from build123d import *

# Parameters (mm, degrees)
F1_DEPTH = 3
F2_W     = 261
F2_H     = 166
F2_R     = 3
F3_DEPTH = 3
F4_R     = 4.99999


# Not quite as in the source:
# - a fillet or chamfer is up to 0.001 mm smaller than in the source, because OpenCascade refuses the exact size


with BuildPart() as f1:
    # F0 (on Front) → F1 (new body)
    with BuildSketch(Plane.XZ):
        Polygon((170, -120), (170, 120), (-170, 120), (-170, -120), (-165, -120), (-165, -110), (-159.5, -110), (-159.5, -120), (159.5, -120), (159.5, -110), (165, -110), (165, -120), align=None)
    extrude(amount=F1_DEPTH)

    # F2 (on face) → F3 (cut, through all)
    with BuildSketch(Plane.XZ.offset(3)):
        Rectangle(F2_W, F2_H)
        with Locations((0, -112)):
            Circle(F2_R)
    extrude(amount=-F3_DEPTH, mode=Mode.SUBTRACT)

    # F4 (radius 5 in the source; OpenCascade refuses exactly that, so slightly less here)
    f4_edges = [f1.edges().sort_by_distance(p)[0] for p in [
        (-170, -1.5, 120),
        (170, -1.5, 120),
        (170, -1.5, -120),
        (-170, -1.5, -120),
    ]]
    fillet(f4_edges, radius=F4_R)


solid = f1.part
For this review, take the finished solid that the model builds, in its own axes (mm). Round coordinates to 2 decimals unless told otherwise and drop trailing zeros. Write each loop counter-clockwise with the first axis right and the second up, starting at its lowest first coordinate (ties: lowest second). Pieces come first, ordered by that corner, then holes. Notation, with made-up numbers: M 71,73 L 91,73 A19 cw 91,103 Z; hole C 80.25,10.5 d8. An arc over 180 degrees is marked long. Write item = value, one per line. Start each with the question number.
(1) We need section B-B (z = -57). Give the boundary of the cut face in (x, y).
(2) We need section C-C (y = -0.6). Give the number of separate pieces and of enclosed holes in the cut face, then the cut area to 3 significant figures.
(3) Clearance check with flat-ended pins moving along their axes: pin 1 Ø1.5 at (x, y) = (161.5, -1) entering from -Z; pin 2 Ø0.9 at (y, z) = (-1.5, -117) entering from +X; pin 3 Ø5 at (x, z) = (0, -112) entering from -Y (1 decimal); pin 4 Ø0.9 at (y, z) = (-1.5, -115.5) entering from -X. State where each tip first meets the part, or that it passes through.
(4) We need section A-A (x = -16.5). Give the boundary of the cut face in (y, z).
(5) For line 1 along Z through (x, y) = (0, -1.15); line 2 along Z through (x, y) = (70, -1.9); line 3 along X through (y, z) = (-1.05, 34.5), list the stretches that pass through material, from the lowest coordinate up.
Results found:
q1.outline = M -170,-3 L -130.5,-3 L -130.5,0 L -170,0 Z; M 130.5,-3 L 170,-3 L 170,0 L 130.5,0 Z
q2.separate_pieces = 1
q2.enclosed_holes = 2
q2.area = 38,100 mm²
q3.pin_1 = -110
q3.pin_2 = 169.75
q3.pin_3 = through
q3.pin_4 = -170
q4.outline = M -3,-120 L 0,-120 L 0,-83 L -3,-83 Z; M -3,83 L 0,83 L 0,120 L -3,120 Z
q5.line_1 = -120 to -115, -109 to -83, 83 to 120
q5.line_2 = -120 to -83, 83 to 120
q5.line_3 = -170 to -130.5, 130.5 to 170
